Verification items for the finished model (mm, model axes). Face numbers are marked on the shaded views. A direction names the side the tool comes from. Coordinates: 2 decimals unless noted, no trailing zeros. Order: outer loops, then holes, each group sorted by start corner. A loop starts at its lowest first (then second) coordinate and runs counter-clockwise, first axis right, second up. Notation, with made-up numbers: (-37.75, 19.25) - (-15.75, 19.25) arc R27 ccw to (-15.75, 55.25) - close; hole circle Ø9 at (-9, 76.5). An arc over 180 degrees is marked (long way). One line per question, with ' | ' between items. Start each with the question number.
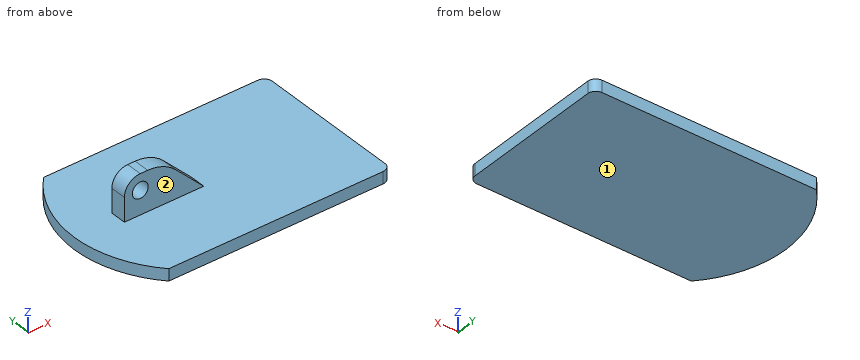
from build123d import *

# Parameters (mm, degrees)
F0_W      = 28
F0_H      = 20
F1_DEPTH  = 1.5
F2_R      = 1
F3_W      = 10
F3_H      = 1
F4_DEPTH  = 5
F5_R      = 2
F6_SIZE   = 4.99999
F7_R      = 5
F9_R      = 1
F10_DEPTH = 25
F12_DEPTH = 1.5


# Not quite as in the source:
# - a fillet or chamfer is up to 0.001 mm smaller than in the source, because OpenCascade refuses the exact size


with BuildPart() as f1:
    # F0 (on Top) → F1 (new body)
    with BuildSketch(Plane.XY):
        Rectangle(F0_W, F0_H)
    extrude(amount=F1_DEPTH)

    # F2
    f2_edges = [f1.edges().sort_by_distance(p)[0] for p in [
        (14, -10, 0.75),
        (14, 10, 0.75),
    ]]
    fillet(f2_edges, radius=F2_R)



with BuildPart() as f4:
    # F3 (on face) → F4 (new body)
    with BuildSketch(Plane.XY.offset(1.5)):
        with Locations((-7.5, 0.5)):
            Rectangle(F3_W, F3_H)
    extrude(amount=F4_DEPTH)

    # F5
    f5_edges = [f4.edges().sort_by_distance(p)[0] for p in [
        (-12.5, 0.5, 6.5),
    ]]
    fillet(f5_edges, radius=F5_R)

    # F6 (size 5 in the source; OpenCascade refuses exactly that, so slightly less here)
    f6_edges = [f4.edges().sort_by_distance(p)[0] for p in [
        (-2.5, 0.5, 6.5),
    ]]
    chamfer(f6_edges, length=F6_SIZE)

    # F7
    f7_edges = [f4.edges().sort_by_distance(p)[0] for p in [
        (-7.49999, 0.5, 6.5),
    ]]
    fillet(f7_edges, radius=F7_R)


with BuildPart() as f1_1:
    add(f1.part)

    add(f4.part)  # F8 merges F4
    # F8: F4 across plane
    add(f4.part.mirror(Plane.XZ))

    # F9 (on face) → F10 (cut)
    with BuildSketch(Plane.XZ.offset(1)):
        with Locations((-10.5, 4.5)):
            Circle(F9_R)
    extrude(amount=-F10_DEPTH, mode=Mode.SUBTRACT)

    # F11 (on face) → F12 (join)
    with BuildSketch(Plane(origin=(0, 0, 0), x_dir=(1, 0, 0), z_dir=(0, 0, -1))):
        with BuildLine():
            Line((-14, -10), (-14, 10))
            ThreePointArc((-14, 10), (-18, 0), (-14, -10))
        make_face()
    extrude(amount=-F12_DEPTH)


solid = f1_1.part
Item 1: Section check A-A (z = 0.5). Record the cut outline in (x, y).
Item 2: Set-up check for the marked faces 1 and 2: record each of +Z, -Z, +X, -X, +Y, -Y from which the full face is reachable in a straight line by a thin tool's end or side.
Item 3: Gauge pin test, flat ends, axial feed: pin 1 (1.5 mm diameter, centred on x = -9, z = 4, fed in from +Y); pin 2 (1 mm diameter, centred on x = 8.5, z = 2.5, fed in from +Y); pin 3 (2.5 mm diameter, centred on x = -7, z = 5, fed in from -Y); pin 4 (1.6 mm diameter, centred on y = -0.5, z = 3, fed in from -X). Record the tip position at first contact, or that the pin passes through.
Item 4: Section check B-B (x = -9). Record the cut outline in (y, z).
Item 5: Section check C-C (y = 5.5). Record the cut outline in (x, z), then the cut area to 3 significant figures.
Item 6: Section check D-D (x = -4). Record the cut outline in (y, z).
Item 7: Thickness scan on probe 1 along Z at (x, y) = (-10.5, -0.3); probe 2 along Z at (x, y) = (1.5, -8); probe 3 along Y at (x, z) = (-7.5, 4.25). Record the ranges inside material, lowest first. Write a range as from..to.
Completed:
1) outline: (-14, -10) - (13, -10) arc R1 ccw to (14, -9) - (14, 9) arc R1 ccw to (13, 10) - (-14, 10) arc R14.5 ccw to start
2) face 1: -Z, +X, -X, +Y, -Y | face 2: +Z, +X, -X, -Y
3) pin 1: stops at y = 1 | pin 2: passes through | pin 3: stops at y = -1 | pin 4: stops at x = -12.5
4) outline: (-10, 0) - (10, 0) - (10, 1.5) - (1, 1.5) - (1, 6.47) - (-1, 6.47) - (-1, 1.5) - (-10, 1.5) - close
5) outline: (-16.92, 0) - (14, 0) - (14, 1.5) - (-16.92, 1.5) - close | area: 46.4 mm^2
6) outline: (-10, 0) - (10, 0) - (10, 1.5) - (1, 1.5) - (1, 3) - (-1, 3) - (-1, 1.5) - (-10, 1.5) - close
7) probe 1: z = 0..3.5, 5.5..6.5 | probe 2: z = 0..1.5 | probe 3: y = -1..1
